Print and shaded views of the part. All mm, measured from the part's lowest x, y and z. Coordinates: 2 decimals unless noted, no trailing zeros. Order: outer loops, then holes, each group sorted by start corner. A loop starts at its lowest first (then second) coordinate and runs counter-clockwise, first axis right, second up.
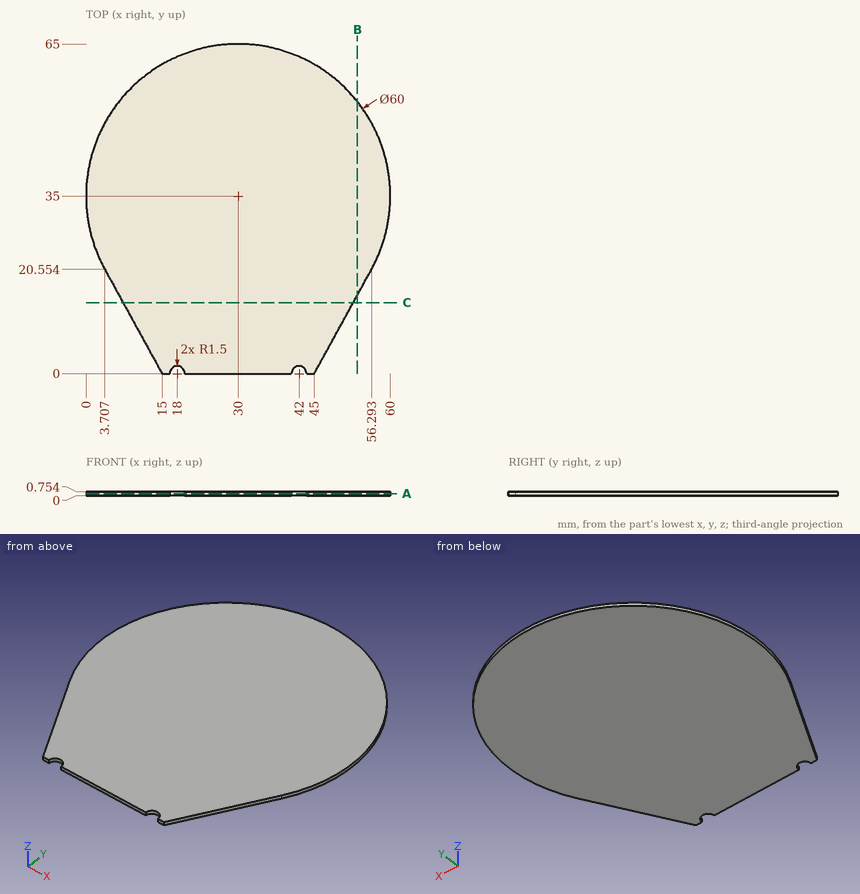
Q1. Probe line 1 (X direction, y = 24.5, z = 0.45); line 2 (X direction, y = 26, z = 0.3); line 3 (Y direction, x = 32, z = 0.6). List the from-to ranges inside material, lowest first.
Established:
line 1: x = 1.9 to 58.1
line 2: x = 1.38 to 58.62
line 3: y = 0 to 64.93
Q2. Cut at C-C, the plane y = 14. List the corners of the cut face in (x, z) (1 decimal).
Established:
outline: (7.3, 0) - (52.7, 0) - (52.7, 0.8) - (7.3, 0.8) - close
Q3. Cut at B-B, the plane x = 53.5. List the corners of the cut face in (y, z) (1 decimal).
Established:
outline: (15.5, 0) - (53.6, 0) - (53.6, 0.8) - (15.5, 0.8) - close
Q4. Cut at A-A, the plane z = 0.35. List the corners of the cut face in (x, y), plus the area to 3 significant figures.
Established:
outline: (3.71, 20.55) - (15, 0) - (16.5, 0) arc R1.5 cw to (19.5, 0) - (40.5, 0) arc R1.5 cw to (43.5, 0) - (45, 0) - (56.29, 20.55) arc R30 ccw (long way) to start
area: 3,090 mm2
